from build123d import *

# Parameters (mm, degrees)
F1_DEPTH = 25
F3_DEPTH = 2.5
F4_R     = 2.5


with BuildPart() as f1:
    # F0 (on Right) → F1 (new body)
    with BuildSketch(Plane.YZ):
        Polygon((0, 0), (0, 23), (-2.5, 23), (-2.5, 3), (-7.5, 3), (-7.5, 14), (-25, 6.5), (-25, 0), align=None)
    extrude(amount=F1_DEPTH)

    # F2 (on face) → F3 (cut, through all)
    with BuildSketch(Plane(origin=(0, 0, 0), x_dir=(-1, 0, 0), z_dir=(0, 1, 0))):
        Polygon((-25, 23), (-25, 3), (-20.25, 3), (-20.25, 22.99), (-15.75, 22.99), (-15.75, 3), (-12.5, 3), (-9.25, 3), (-9.25, 22.99), (-4.75, 22.99), (-4.75, 3), (0, 3), (0, 23), align=None)
    extrude(amount=-F3_DEPTH, mode=Mode.SUBTRACT)

    # F4
    f4_edges = [f1.edges().sort_by_distance(p)[0] for p in [
        (20.25, -1.25, 3),
        (18, -2.5, 3),
        (7, -2.5, 3),
        (9.25, -1.25, 3),
        (15.75, -1.25, 3),
        (4.75, -1.25, 3),
    ]]
    fillet(f4_edges, radius=F4_R)


solid = f1.part
Model file for the job. Use its own axes, mm. A direction names the side the tool comes from. Give positions to 0.01 mm unless a question says otherwise; leave off trailing zeros. Order: outer loops, then holes, each group sorted by start corner. A loop starts at its lowest first (then second) coordinate and runs counter-clockwise, first axis right, second up. Notation, with made-up numbers: (56.5, -33) -> (66.5, -33) arc R31 cw to (66.5, -2) -> close; hole circle Ø8 at (68, 28). An arc over 180 degrees is marked (long way). Use CSV: the item, a comma, the result in double quotes.
1. Band-saw the part on B-B, the plane x = 8.5. Give the cut face in (y, z).
Outcome:
outline,"(-25, 0) -> (0, 0) -> (0, 22.99) -> (-2.5, 22.99) -> (-2.5, 5.5) arc R2.5 cw to (-5, 3) -> (-7.5, 3) -> (-7.5, 14) -> (-25, 6.5) -> close"
2. Drill centre lines: line 1 along X through (y, z) = (-2.25, 19.75); line 2 along Y through (x, z) = (16.75, 21.5); line 3 along Y through (x, z) = (9.75, 6). Where is each one in solid material? Low to high. Write a range as from..to.
Outcome:
line 1,"4.75..9.25, 15.75..20.25"
line 2,"-2.5..0"
line 3,"-25..-7.5"
3. Drop flat-ended pins along their axis: pin 1 (2 mm diameter, centred on x = 13.5, y = -5.5, fed in from +Z); pin 2 (3 mm diameter, centred on x = 12, y = -14.5, fed in from +Z); pin 3 (1 mm diameter, centred on x = 9.5, y = -13.5, fed in from -Z); pin 4 (5 mm diameter, centred on x = 6.5, z = 12.5, fed in from -Y). Give the stop position or say it passes through.
Outcome:
pin 1,"z = 3.05"
pin 2,"z = 11.64"
pin 3,"z = 0"
pin 4,"y = -16.83"
4. Band-saw the part on C-C, the plane z = 8.25. Give the cut face in (x, y).
Outcome:
outline,"(0, -20.92) -> (25, -20.92) -> (25, -7.5) -> (0, -7.5) -> close; (4.75, -2.5) -> (9.25, -2.5) -> (9.25, 0) -> (4.75, 0) -> close; (15.75, -2.5) -> (20.25, -2.5) -> (20.25, 0) -> (15.75, 0) -> close"
5. Band-saw the part on A-A, the plane z = 20.25. Give the cut face in (x, y), then the cut area to 3 significant figures.
Outcome:
outline,"(4.75, -2.5) -> (9.25, -2.5) -> (9.25, 0) -> (4.75, 0) -> close; (15.75, -2.5) -> (20.25, -2.5) -> (20.25, 0) -> (15.75, 0) -> close"
area,"22.5 mm²"
6. Band-saw the part on D-D, the plane y = -1.25. Give the cut face in (x, z).
Outcome:
outline,"(0, 0) -> (25, 0) -> (25, 3) -> (22.75, 3) arc R2.5 cw to (20.25, 5.5) -> (20.25, 22.99) -> (15.75, 22.99) -> (15.75, 5.5) arc R2.5 cw to (13.25, 3) -> (11.75, 3) arc R2.5 cw to (9.25, 5.5) -> (9.25, 22.99) -> (4.75, 22.99) -> (4.75, 5.5) arc R2.5 cw to (2.25, 3) -> (0, 3) -> close"
7. 3-axis set-ups, long thin cutter, end or side, ignore diameter. For faces 1 (the cylindrical face through (3.71, -1.98, 3.47)), 2 (the flat face through (13, -5, 3)), 3 (the flat face through (12, -7.5, 8)), 4 (the cylindrical face through (21.29, -1.98, 3.47)), 5 (the cylindrical face through (14.71, -1.98, 3.47)): which of +Z, -Z, +X, -X, +Y, -Y reach the whole face in a straight line?
Outcome:
face 1,"+Z, -X, +Y"
face 2,"+Z"
face 3,"+Z, +X, -X"
face 4,"+Z, +X, +Y"
face 5,"+Z, +Y"
